Here's how the part is built. I have some questions about the finished solid (model axes, mm). Face numbers are marked on the shaded views. Give positions to 0.01 mm unless a question says otherwise; leave off trailing zeros. Write each loop counter-clockwise with the first axis right and the second up, starting at its lowest first coordinate (ties: lowest second). Pieces come first, ordered by that corner, then holes. Notation, with made-up numbers: (69.5, 28.25) -> (108.5, 28.25) arc R24 ccw to (108.5, 50.25) -> close; hole circle Ø6 at (49.25, 12.5). An arc over 180 degrees is marked (long way). Use CSV: the item, a comma, the result in double quotes. Start each with the question number.
(1) Suppose I cut it at C-C on z = 1276. List the corners of the cut face in (x, y) for me.
(2) I need wall thicknesses on L1, parallel to Z at x = 15.5, y = 147; L2, parallel to Y at x = 16, z = 1329; L3, parallel to Z at x = 14.5, y = 173.5. Which ranges of each line are inside material? Lowest first, please. Write a range as [from, to].
(3) For pin 1 Ø11.5 at (y, z) = (195.7, 1328.48) entering from -X; pin 2 Ø2 at (x, z) = (14, 1320) entering from +Y; pin 3 Ø1.5 at (x, y) = (15, 155) entering from -Z; pin 4 Ø1.9 at (x, z) = (14, 1321.5) entering from -Y, each with a flat end and sliding along its axis, tell me the tip position at first contact or that it passes through.
(4) Suppose I cut it at B-B on x = 15. Give the number of separate pieces and of enclosed holes in the cut face, plus the area to 3 significant figures.
(5) If we mould it in two halves opening along Z, with no side actions, what happens to the marked faces 1, 2, 3 and 4? For each: pulls with the +Z half, pulls with the -Z half, needs draft (parallel to the pull), parting line crosses it, or undercut.
(6) Suppose I cut it at A-A on z = 1305. List the corners of the cut face in (x, y) for me, plus the area to 3 significant figures.
(7) Suppose I cut it at D-D on y = 163. List the corners of the cut face in (x, z) for me.
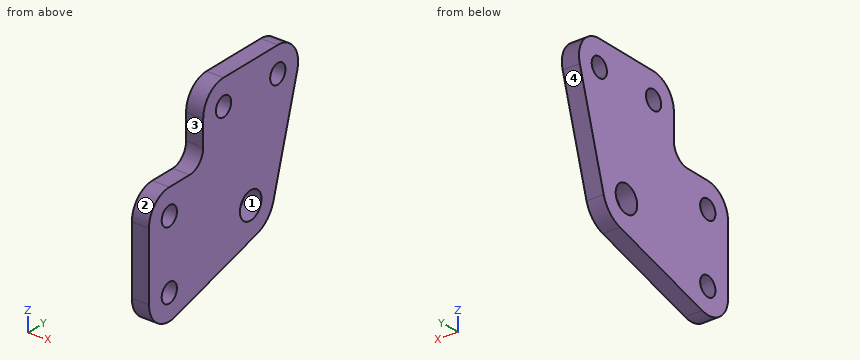
from build123d import *

# Parameters (mm, degrees)
BOSS_EXTRUDE1_START     = 12.388912
BOSS_EXTRUDE1_DEPTH     = 6.35
F_3_8_CLEARANCE_HOLE1_D = 10.0838
F_1_4_CLEARANCE_HOLE1_D = 7.14248
FILLET1_R               = 6.35


with BuildPart() as part:
    # Sketch1 → Boss-Extrude1 (new body)
    with BuildSketch(Plane(origin=(0, 0, 0), x_dir=(0, 0, -1), z_dir=(1, 0, 0)).offset(BOSS_EXTRUDE1_START)):
        with BuildLine():
            Line((-1338.000334154, 195.704574554), (-1338.000334154, 170.304574554))
            ThreePointArc((-1338.000334154, 170.304574554), (-1335.210526245, 163.569382463), (-1328.475334154, 160.779574554))
            Line((-1328.475334154, 160.779574554), (-1312.600334154, 160.779574554))
            Line((-1312.600334154, 160.779574554), (-1312.600334154, 144.904574554))
            ThreePointArc((-1312.600334154, 144.904574554), (-1309.810526245, 138.169382463), (-1303.075334154, 135.379574554))
            Line((-1303.075334154, 135.379574554), (-1277.675334154, 135.379574554))
            ThreePointArc((-1277.675334154, 135.379574554), (-1270.059858037, 139.183547679), (-1268.527125538, 147.557102426))
            Line((-1268.527125538, 147.557102426), (-1279.702424102, 186.099190405))
            ThreePointArc((-1279.702424102, 186.099190405), (-1282.517610048, 190.86229866), (-1287.280718303, 193.677484606))
            Line((-1287.280718303, 193.677484606), (-1325.822806282, 204.85278317))
            ThreePointArc((-1325.822806282, 204.85278317), (-1334.196361029, 203.320050671), (-1338.000334154, 195.704574554))
        make_face()
    extrude(amount=BOSS_EXTRUDE1_DEPTH)

    # 3/8 Clearance Hole1 (through all)
    with Locations(Plane(origin=(18.738912484, 0, 0), x_dir=(0, 0, -1), z_dir=(1, 0, 0))):
        with Locations((-1290.375334154, 183.004574554)):
            Hole(F_3_8_CLEARANCE_HOLE1_D / 2)

    # 1/4 Clearance Hole1 (through all)
    with Locations(Plane(origin=(18.738912484, 0, 0), x_dir=(0, 0, -1), z_dir=(1, 0, 0))):
        with Locations((-1303.075334154, 144.904574554), (-1277.675334154, 144.904574554), (-1328.475334154, 170.304574554), (-1328.475334154, 195.704574554)):
            Hole(F_1_4_CLEARANCE_HOLE1_D / 2)

    # Fillet1
    fillet1_edges = [part.edges().sort_by_distance(p)[0] for p in [
        (15.563912, 160.779574554, 1312.600334154),
    ]]
    fillet(fillet1_edges, radius=FILLET1_R)


solid = part.part
Geometry says:
1,outline,"(12.39, 135.53) -> (18.74, 135.53) -> (18.74, 141.75) -> (12.39, 141.75) -> close; (12.39, 148.06) -> (18.74, 148.06) -> (18.74, 173.33) -> (12.39, 173.33) -> close"
2,L1,"[1268.38, 1274.78], [1280.57, 1300.18], [1305.97, 1312.6]"
2,L2,"[160.79, 166.77], [173.84, 192.17], [199.24, 205.22]"
2,L3,"[1276.05, 1326.88], [1330.07, 1338]"
3,pin 1,"x = 12.39"
3,pin 2,"y = 203.45"
3,pin 3,"z = 1270.47"
3,pin 4,"y = 160.78"
4,separate pieces,"1"
4,enclosed holes,"5"
4,area,"3,140 mm²"
5,face 1,"undercut"
5,face 2,"pulls with the +Z half"
5,face 3,"needs draft"
5,face 4,"pulls with the -Z half"
6,outline,"(12.39, 135.58) -> (18.74, 135.58) -> (18.74, 141.9) -> (12.39, 141.9) -> close; (12.39, 147.91) -> (18.74, 147.91) -> (18.74, 198.82) -> (12.39, 198.82) -> close"
6,area,"363 mm²"
7,outline,"(12.39, 1273) -> (18.74, 1273) -> (18.74, 1334.59) -> (12.39, 1334.59) -> close"
